Verification items for the finished model (mm, model axes). A direction names the side the tool comes from. Coordinates: 2 decimals unless noted, no trailing zeros. Order: outer loops, then holes, each group sorted by start corner. A loop starts at its lowest first (then second) coordinate and runs counter-clockwise, first axis right, second up. Notation, with made-up numbers: (-19.75, -30) -> (-8.75, -30) arc R11 ccw to (-8.75, -12) -> close; hole circle Ø10 at (-33, -38). An arc over 180 degrees is marked (long way). Write each question's results on one line, items separated by ' | '. Start each with the question number.
(1) Thickness scan on probe 1 along X at (y, z) = (5, -70); probe 2 along Z at (x, y) = (3, 5.5); probe 3 along Y at (x, z) = (1.5, -65). Record the ranges inside material, lowest first. Write a range as [from, to].
(2) Set-up check for faces 1 (the flat face through (3, 0, -5)), 2 (the cylindrical face through (1.97, 51.15, -63.5)): record each of +Z, -Z, +X, -X, +Y, -Y from which the full face is reachable in a straight line by a thin tool's end or side.
(3) Cross-section at A-A on y = 102. Enter the section's corners in (x, z), and give its area (3 significant figures).
(4) Cross-section at B-B on z = -6. Enter the section's corners in (x, y).
(5) Draft check along Y on faces 3 (the cylindrical face through (3.04, 3.61, -10.44)), 4 (the flat face through (1.97, 58.78, -84.87)), 5 (the cylindrical face through (2.028, 81.602, -78.394)), 6 (the flat face through (1.97, 101.47, -50.22)). Enter one of: +Y half, -Y half, draft (parallel to the pull), parting line (faces both ways), or undercut.
(6) Go/stop test with flat-tipped pins: pin 1 (2 mm diameter, centred on x = 4, z = -82.5, fed in from +Y); pin 2 (3 mm diameter, centred on x = 0.5, y = 81, fed in from +Z); pin 3 (3 mm diameter, centred on x = 2, y = 52, fed in from -Z). Record where each tip stops, or that it passes through.
```python
from build123d import *

# Parameters (mm, degrees)
SKETCH1_R                   = 1.5
BOSS_EXTRUDE1_DEPTH         = 6
FILLET1_R                   = 3
TAP_DRILL_FOR_M3_TAP1_D     = 2.5
TAP_DRILL_FOR_M3_TAP1_DEPTH = 8
TAP_DRILL_FOR_M3_TAP1_TIP   = 0.751075774
CUT_EXTRUDE1_START          = -2
CUT_EXTRUDE1_DEPTH          = 2
CUT_EXTRUDE2_REACH          = 147.011
SKETCH7_R                   = 1.5


with BuildPart() as part:
    # Sketch1 → Boss-Extrude1 (new body)
    with BuildSketch(Plane(origin=(0, 0, 0), x_dir=(0, 0, -1), z_dir=(1, 0, 0))):
        with BuildLine():
            Line((0, 0), (0, 6))
            Line((0, 6), (36.541818306, 22.269465723))
            ThreePointArc((36.541818306, 22.269465723), (55.71908903, 43.197784292), (53.491952961, 71.496231166))
            Line((53.491952961, 71.496231166), (40.346749203, 96.218763766))
            Line((40.346749203, 96.218763766), (62.341129166, 107.913383036))
            Line((62.341129166, 107.913383036), (87.292806812, 82.883380245))
            ThreePointArc((87.292806812, 82.883380245), (88.459285656, 79.986445673), (87.187944242, 77.133974145))
            ThreePointArc((87.187944242, 77.133974145), (85.791082043, 75.901173525), (84.328789644, 74.746737597))
            Line((84.328789644, 74.746737597), (95.922273052, 48.707347523))
            Line((95.922273052, 48.707347523), (98.362692911, 43.226074777))
            ThreePointArc((98.362692911, 43.226074777), (82.081212508, 29.320376834), (76, 8.790547467))
            Line((76, 8.790547467), (76, 0))
            Line((76, 0), (66, 0))
            Line((66, 0), (66, 3.884469182))
            ThreePointArc((66, 3.884469182), (38, 10.818472536), (10, 3.884469182))
            Line((10, 3.884469182), (10, 0))
            Line((10, 0), (0, 0))
        make_face()
        with Locations((64, 102)):
            Circle(SKETCH1_R, mode=Mode.SUBTRACT)
        with BuildLine():
            Line((78.174939554, 34.237907891), (39.032120003, 16.810401803))
            ThreePointArc((39.032120003, 16.810401803), (55.025629399, 14.584670036), (70, 8.541951295))
            Line((70, 8.541951295), (70, 8.790547467))
            ThreePointArc((70, 8.790547467), (72.093906618, 22.154657887), (78.174939554, 34.237907891))
        make_face(mode=Mode.SUBTRACT)
        with BuildLine():
            Line((56.201627065, 31.02257653), (90.441000307, 46.266927665))
            Line((90.441000307, 46.266927665), (79.173694043, 71.573711875))
            ThreePointArc((79.173694043, 71.573711875), (75.490729324, 70.000575949), (71.648335848, 68.871417797))
            Line((71.648335848, 68.871417797), (61.936537439, 66.629272466))
            ThreePointArc((61.936537439, 66.629272466), (63.129066114, 48.17201256), (56.201627065, 31.02257653))
        make_face(mode=Mode.SUBTRACT)
        with BuildLine():
            Line((80.108700039, 81.591428686), (61.231449963, 100.527935833))
            Line((61.231449963, 100.527935833), (48.461264136, 93.737907585))
            Line((48.461264136, 93.737907585), (58.884294031, 74.135039414))
            Line((58.884294031, 74.135039414), (69.848727413, 76.666378316))
            ThreePointArc((69.848727413, 76.666378316), (75.251497028, 78.560635362), (80.108700039, 81.591428686))
        make_face(mode=Mode.SUBTRACT)
        with BuildLine():
            ThreePointArc((71.085958212, 71.307342959), (78.788354228, 74.187150825), (85.482948342, 78.962358399))
            ThreePointArc((85.482948342, 78.962358399), (85.556981354, 81.082386492), (83.436953262, 81.156419504))
            ThreePointArc((83.436953262, 81.156419504), (77.379939539, 76.835993604), (70.411105049, 74.230453154))
            ThreePointArc((70.411105049, 74.230453154), (69.286976533, 72.431471475), (71.085958212, 71.307342959))
        make_face(mode=Mode.SUBTRACT)
    extrude(amount=BOSS_EXTRUDE1_DEPTH)

    # Fillet1
    fillet1_edges = [part.edges().sort_by_distance(p)[0] for p in [
        (3, 3.884469182, -66),
        (3, 3.884469182, -10),
        (3, 43.226074777, -98.362692911),
        (3, 16.810401803, -39.032120003),
        (3, 34.237907891, -78.174939554),
        (3, 8.541951295, -70),
        (3, 46.266927665, -90.441000307),
        (3, 31.02257653, -56.201627065),
        (3, 81.591428686, -80.108700039),
        (3, 107.913383036, -62.341129166),
        (3, 100.527935833, -61.231449963),
        (3, 93.737907585, -48.461264136),
        (3, 74.135039414, -58.884294031),
        (3, 6, 0),
        (3, 66.629272466, -61.936537439),
        (3, 74.746737597, -84.328789644),
        (3, 71.573711875, -79.173694043),
    ]]
    fillet(fillet1_edges, radius=FILLET1_R)

    # Tap Drill for M3 Tap1
    with Locations(Plane(origin=(0, 0, 0), x_dir=(-1, 0, 0), z_dir=(0, -1, 0))):
        with Locations((-3, 3), (-3, 70)):
            Hole(TAP_DRILL_FOR_M3_TAP1_D / 2, depth=TAP_DRILL_FOR_M3_TAP1_DEPTH)
            with Locations((0, 0, -(TAP_DRILL_FOR_M3_TAP1_DEPTH + TAP_DRILL_FOR_M3_TAP1_TIP / 2))):  # 118° drill point
                Cone(0, TAP_DRILL_FOR_M3_TAP1_D / 2, TAP_DRILL_FOR_M3_TAP1_TIP, mode=Mode.SUBTRACT)

    # Sketch6 → Cut-Extrude1 (cut)
    with BuildSketch(Plane(origin=(6, 0, 0), x_dir=(0, 0, -1), z_dir=(1, 0, 0)).offset(CUT_EXTRUDE1_START)):
        with BuildLine():
            Line((0, 6), (0, 120))
            Line((0, 120), (100, 120))
            Line((100, 120), (100, 4.781422789))
            Line((100, 4.781422789), (76, 4.781422789))
            ThreePointArc((76, 4.781422789), (42.323682099, 16.676697331), (7.381236086, 9.286338039))
            Line((7.381236086, 9.286338039), (0, 6))
        make_face()
    extrude(amount=CUT_EXTRUDE1_DEPTH, mode=Mode.SUBTRACT)

    # Sketch7 → Cut-Extrude2 (cut, up to next)
    with BuildSketch(Plane(origin=(6, 0, 0), x_dir=(0, 0, -1), z_dir=(1, 0, 0)), mode=Mode.PRIVATE) as cut_extrude2_sk1:
        with Locations((14.009846336, 8.95367663)):
            Circle(SKETCH7_R)
    cut_extrude2_tool1 = extrude(cut_extrude2_sk1.sketch, amount=-CUT_EXTRUDE2_REACH, mode=Mode.PRIVATE) & part.part
    # Sketch7 → Cut-Extrude2 (cut, up to next)
    with BuildSketch(Plane(origin=(6, 0, 0), x_dir=(0, 0, -1), z_dir=(1, 0, 0)), mode=Mode.PRIVATE) as cut_extrude2_sk2:
        with Locations((93.488301151, 44.339764578)):
            Circle(SKETCH7_R)
    cut_extrude2_tool2 = extrude(cut_extrude2_sk2.sketch, amount=-CUT_EXTRUDE2_REACH, mode=Mode.PRIVATE) & part.part
    add(cut_extrude2_tool1.solids().sort_by_distance((6, 8.953677, -14.009846))[0], mode=Mode.SUBTRACT)
    add(cut_extrude2_tool2.solids().sort_by_distance((6, 44.339765, -93.488301))[0], mode=Mode.SUBTRACT)


solid = part.part
```
Results are:
1) probe 1: x = [0, 1.75], [4.25, 6] | probe 2: z = [-76, -71.25], [-68.75, -62.7], [-13.3, -4.25], [-1.75, -0.37] | probe 3: y = [4.28, 11.04], [28.37, 34.94], [67.34, 75.55], [96.75, 100.88], [103.12, 105.25]
2) face 1: +Z, -Z, +X, -X, -Y | face 2: +X, -X
3) outline: (0, -68.24) -> (4, -68.24) -> (4, -65.5) -> (0, -65.5) -> close; (0, -62.5) -> (4, -62.5) -> (4, -51.22) -> (0, -51.22) -> close | area: 56.1 mm2
4) outline: (0, 0) -> (6, 0) -> (6, 8.67) -> (0, 8.67) -> close
5) face 3: -Y half | face 4: undercut | face 5: undercut | face 6: +Y half
6) pin 1: stops at y = 88.69 | pin 2: stops at z = -47.64 | pin 3: stops at z = -95.12
